Autodesk Inventor part; units mm, degrees
ref_plane "Work Plane2" through (-125.0759, -150, 0) normal (0, 0, 1) x (1, 0, 0)
ref_plane "Work Plane3" through (-125.0759, -150, 0) normal (0, 0, 1) x (1, 0, 0)
ref_plane "YZ Plane" through (0, 0, 0) normal (1, 0, 0) x (0, 1, 0)
ref_plane "Work Plane1" through (0, 0, 0) normal (0, 0, 1) x (1, 0, 0)
sketch "Sketch1" plane through (0, 0, 0) normal (0, 0, 1) x (1, 0, 0)
  line L0 (0, -150) -> (-125.0759, -150)
  line L1 (0, 0) -> (0, -150)
  line L2 (-125.0759, 0) -> (0, 0)
  line L3 (-125.0759, 0) -> (-125.0759, -150)
  line L4 (-5, -147.5) -> (-117.0759, -147.5)
  line L5 (-117.0759, -147.5) -> (-117.0759, -2.5)
  line L6 (-117.0759, -2.5) -> (-5, -2.5)
  line L7 (-5, -2.5) -> (-5, -147.5)
  line L8 (0, -150) -> (-125.0759, -150)
  line L9 (0, 0) -> (0, -150)
  line L10 (-125.0759, 0) -> (0, 0)
  line L11 (-125.0759, 0) -> (-125.0759, -150)
  line L12 (-5, -147.5) -> (-117.0759, -147.5)
  line L13 (-117.0759, -147.5) -> (-117.0759, -2.5)
  line L14 (-117.0759, -2.5) -> (-5, -2.5)
  line L15 (-5, -2.5) -> (-5, -147.5)
  line L16 (-5, -2.5) -> (0, -2.5)
  line L17 (-5, -147.5) -> (0, -147.5)
  line L18 (-5, -2.5) -> (-10, -2.5)
  line L19 (-10, -2.5) -> (-10, -7.5)
  line L20 (-10, -7.5) -> (-5, -7.5)
  line L21 (-5, -7.5) -> (-5, -2.5)
  line L22 (-5, -147.5) -> (-10, -147.5)
  line L23 (-10, -147.5) -> (-10, -142.5)
  line L24 (-10, -142.5) -> (-5, -142.5)
  line L25 (-5, -142.5) -> (-5, -147.5)
  dimension "d2" = 5
  dimension "d3" = 5
  dimension "d4" = 5
  dimension "d5" = 5
extrude "Extrusion1" add sketch "Sketch1" along normal blind 250 contours L0 L3 L2 L1 L16 L6 L5 L4 L17 | L4 L23 L24 L7 | L7 L20 L19 L6
sketch "Sketch2" plane through (0, 0, 250) normal (0, 0, 1) x (1, 0, 0)
  line L0 (-5, -2.5) -> (-2, -2.5)
  line L1 (-2, -2.5) -> (-2, -7.5)
  line L2 (0, -2.5) -> (-2, -2.5)
  line L3 (-2, -2.5) -> (-2, -7.5)
  line L4 (-2, -7.5) -> (0, -7.5)
  line L5 (0, -7.5) -> (0, -2.5)
  line L6 (-117.0759, -147.5) -> (-117.0759, -2.5)
  line L7 (-117.0759, -75) -> (40.0034, -75) construction
  line L8 (-5, -147.5) -> (-2, -147.5)
  line L9 (-2, -147.5) -> (-2, -142.5)
  line L10 (0, -147.5) -> (-2, -147.5)
  line L11 (-2, -147.5) -> (-2, -142.5)
  line L12 (-2, -142.5) -> (0, -142.5)
  line L13 (0, -142.5) -> (0, -147.5)
  point P0 (0, 0)
ref_plane "Work Plane2" through (-125.0759, -150, 0) normal (0, 0, 1) x (1, 0, 0)
extrude "Extrusion2" add sketch "Sketch2" against normal up to surface (250 mm away)
fillet "Fillet1" radius 2 2 edges at (-5, -142.5, 125) (-5, -7.5, 125)
sketch "Sketch3" plane through (0, 0, 250) normal (0, 0, 1) x (1, 0, 0)
  line L0 (0, -7.5) -> (0, 0)
  line L1 (0, -7.5) -> (-2, -7.5)
  line L2 (-5, -7.5) -> (-5, -142.5)
  line L3 (-2, -142.5) -> (0, -142.5)
  line L4 (0, -142.5) -> (0, -7.5)
  line L5 (-2, -147.5) -> (-2, -142.5)
  line L6 (-2, -147.5) -> (-5, -147.5)
  line L7 (-5, -147.5) -> (-5, -142.5)
  line L8 (-2, -142.5) -> (-2, -147.5)
  line L9 (-5, -2.5) -> (-2, -2.5)
  line L10 (-2, -2.5) -> (-5, -2.5)
  line L11 (-5, -2.5) -> (-5, -7.5)
  line L12 (-2, -7.5) -> (-2, -2.5)
  line L13 (-2, -2.5) -> (-2, -7.5)
  line L14 (-2, -2.7) -> (-5, -2.7)
  line L15 (-2, -147.3) -> (-5, -147.3)
  dimension "d10" = 0.2
  dimension "d11" = 0.2
ref_plane "Work Plane3" through (-125.0759, -150, 0) normal (0, 0, 1) x (1, 0, 0)
properties part number "ForwardSection1" material "Plastic, Opaque White"
Build history of the part. All positions in model axes, mm. A direction names the side the tool comes from. Round coordinates to 2 decimals unless told otherwise and drop trailing zeros. Loops run counter-clockwise (first coordinate to the right, second up) from the corner with the lowest first, then second, coordinate; pieces in that order, holes last.
Item 1: Saw through at B-B (z = 187.5). List the corners of the cut face in (x, y).
Item 2: Saw through at A-A (x = -64). List the corners of the cut face in (y, z).
Item 3: Two-plate mould, pull along Y, no slides. Class faces 3 (the face through (-62, -150, 123)), 4 (the face through (0, -146, 123)), 5 (the face through (-64, -2.5, 123)): released by +Y, released by -Y, zero draft, split by the parting line, or undercut.
Item 4: Which spindle directions (+Z, -Z, +X, -X, +Y, -Y) get a long thin tool onto all of the face, cutting with end or side? Do faces 1 (the face through (-2, -5, 127)), 2 (the face through (0, -4, 123)). Say none if no direction does.
Item 5: Drill centre lines: line 1 along Y through (x, z) = (-20.5, 143.5); line 2 along X through (y, z) = (-13.5, 206.5). Where is each one in solid material? Low to high.
Item 6: Saw through at C-C (y = -69.5). List the corners of the cut face in (x, z).
Item 7: Pin check, flat tip, straight feed: P1, Ø5, axis at x = -51.5, z = 180, coming from the +Y side. Stop position of the tip, or through.
Worked answers:
1. outline: (-125.08, -150) - (0, -150) - (0, -142.5) - (-2, -142.5) - (-2, -147.5) - (-5, -147.5) - (-5, -144.5) arc R2 ccw to (-7, -142.5) - (-10, -142.5) - (-10, -147.5) - (-117.08, -147.5) - (-117.08, -2.5) - (-10, -2.5) - (-10, -7.5) - (-7, -7.5) arc R2 ccw to (-5, -5.5) - (-5, -2.5) - (-2, -2.5) - (-2, -7.5) - (0, -7.5) - (0, 0) - (-125.08, 0) - close
2. outline: (-150, 0) - (-147.5, 0) - (-147.5, 250) - (-150, 250) - close; (-2.5, 0) - (0, 0) - (0, 250) - (-2.5, 250) - close
3. face 3: released by -Y
3. face 4: zero draft
3. face 5: undercut
4. face 1: +Z, -Z
4. face 2: +Z, -Z, +X, +Y, -Y
5. line 1: y = -150 to -147.5, -2.5 to 0
5. line 2: x = -125.08 to -117.08
6. outline: (-125.08, 0) - (-117.08, 0) - (-117.08, 250) - (-125.08, 250) - close
7. P1: stops at y = 0
